Could you check a few things on this model? Use its own coordinates, in mm. A direction names the side the tool comes from. Round coordinates to 2 decimals unless told otherwise and drop trailing zeros. Order: outer loops, then holes, each group sorted by start corner. A loop starts at its lowest first (then second) coordinate and runs counter-clockwise, first axis right, second up. Notation, with made-up numbers: (68, 77.5) -> (106, 77.5) arc R17 ccw to (106, 103.5) -> close; hole circle Ø4 at (32.5, -29). An arc over 180 degrees is marked (long way). One line per question, with ' | ' between items.
Autodesk Inventor part; units mm, degrees
ref_plane "YZ Plane" through (0, 0, 0) normal (1, 0, 0) x (0, 1, 0)
ref_plane "XZ Plane" through (0, 0, 0) normal (0, 1, 0) x (-1, 0, 0)
ref_plane "XY Plane" through (0, 0, 0) normal (0, 0, 1) x (1, 0, 0)
sketch "Sketch1" plane through (0, 0, 0) normal (0, 1, 0) x (-1, 0, 0)
  line L0 (-24, 32.5) -> (24, 32.5)
  line L1 (24, 32.5) -> (24, -32.5)
  line L2 (24, -32.5) -> (-24, -32.5)
  line L3 (-24, -32.5) -> (-24, 32.5)
  line L4 (-24, 32.5) -> (24, -32.5) construction
  line L5 (24, 32.5) -> (-24, -32.5) construction
  line L6 (24, 9.5) -> (-24, 9.5)
  line L7 (-24, 9.5) -> (-24, -32.5)
  line L8 (-24, -32.5) -> (24, -32.5)
  line L9 (24, -32.5) -> (24, 9.5)
  circle A0 centre (0, -11.5) radius 11.25
  line L10 (24, 12.5) -> (-24, 12.5)
  line L11 (-24, 24.95) -> (-24, 20.05)
  line L12 (15.5, -27) -> (-15.5, -27) construction
  line L13 (-15.5, -27) -> (-15.5, 4) construction
  line L14 (-15.5, 4) -> (15.5, 4) construction
  line L15 (15.5, 4) -> (15.5, -27) construction
  line L16 (15.5, -27) -> (-15.5, 4) construction
  line L17 (-15.5, -27) -> (15.5, 4) construction
  line L18 (-24, 52.5) -> (24, 52.5)
  line L19 (24, 52.5) -> (24, 32.5)
  line L20 (24, 32.5) -> (-24, 32.5)
  line L21 (-24, 32.5) -> (-24, 52.5)
  point P0 (0, 0)
  point P1 (-21.1, 9.5)
  point P2 (21.1, 9.5)
  point P3 (18, 42.6936)
  point P4 (-11, 42.5)
  point P5 (18, 22.5)
  point P6 (-11, 22.3064)
  dimension "d0" = 48
  dimension "d1" = 65
  dimension "d2" = 20
  dimension "d3" = 3
  dimension "d4" = 2.9
  dimension "d5" = 2.9
  dimension "d6" = 22.5
  dimension "d35" = 31
  dimension "d36" = 31
  dimension "d71" = 20
  dimension "d73" = 6
  dimension "d74" = 6
  dimension "d82" = 35
  dimension "d83" = 35
extrude "Extrusion1" add sketch "Sketch1" along normal blind 4.2
sketch "Sketch2" plane through (0, 4.2, 0) normal (0, 1, 0) x (1, 0, 0)
  point P0 (0, 0)
  point P1 (11, -42.5)
  point P2 (11, -22.3064)
  point P3 (-18, -22.5)
  point P4 (-18, -42.6936)
hole "Hole5" at (11, 4.2, 42.5) at (-18, 4.2, 42.6936) at (11, 4.2, 22.3064) at (-18, 4.2, 22.5) direction (0, -1, 0) diameter 4.5 end through all
extrude "Extrusion3" add sketch "Sketch1" against normal blind 20 contours L1 L6 L3 L10
sketch "Sketch4" plane through (24, 0, -32.5) normal (1, 0, 0) x (0, 0, -1)
  line L0 (-42, -20) -> (-42, 0)
  line L1 (-42, -20) -> (-22, 0)
  line L2 (0, 0) -> (-42, 0)
  line L3 (-22, 0) -> (-42, 0)
  line L4 (-42, 0) -> (-42, -20)
  point P0 (-32.5, 0)
  dimension "d32" = 20
extrude "Extrusion4" add sketch "Sketch4" against normal blind 2.7
ref_plane "Work Plane1" through (0, 0, 52.5) normal (-1, 0, 0) x (0, 0, 1)
mirror "Mirror1" about plane through (0, 0, 52.5) normal (-1, 0, 0) of "Extrusion4"
sketch "Sketch5" plane through (0, 4.2, 0) normal (0, 1, 0) x (1, 0, 0)
  point P0 (0, 0)
  point P1 (-15.5, 27)
  point P2 (15.5, 27)
  point P3 (-15.5, -4)
  point P4 (15.5, -4)
hole "Hole4" at (-15.5, 4.2, -27) at (15.5, 4.2, -27) at (-15.5, 4.2, 4) at (15.5, 4.2, 4) direction (0, -1, 0) diameter 3.2 depth 8 tip angle 118 countersink diameter 6 countersink angle 90
sketch "Sketch6" plane through (21.3, -20, 9.5) normal (0, 0, -1) x (-1, 0, 0)
  line L0 (42.6, 0) -> (42.6, 20)
  line L1 (0, 20) -> (42.6, 20)
  line L2 (0, 20) -> (0, 0)
  line L3 (42.6, 0) -> (0, 0)
  point P0 (21.3, 20)
extrude "ajustement 0.2mm" cut sketch "Sketch6" against normal blind 0.4
sketch "Sketch7" plane through (0, 4.2, 0) normal (0, 1, 0) x (1, 0, 0)
  circle A0 centre (70.6822, -32.5) radius 55
  line L0 (21.3, -9.9) -> (-21.3, -9.9) construction
  line L1 (21.3, -9.9) -> (21.3, -51.2) construction
  line L2 (137, -22.5) -> (-72, -22.5) construction
  line L3 (0, -123.9517) -> (0, 131.2102) construction
  circle A1 centre (0, 11.5) radius 83.2585 construction
  line L4 (134.8387, -42.5) -> (-75.1613, -42.5) construction
  line L5 (134.8387, -32.5) -> (-75.1613, -32.5) construction
  point P0 (0, 0)
  dimension "d67" = 166.517
  dimension "d53" = 110
  dimension "d69" = 20
  dimension "d70" = 10
sketch "Sketch8" plane through (0, 0, 0) normal (0, -1, 0) x (1, 0, 0)
  line L0 (-21.3, 9.9) -> (21.3, 9.9)
  line L1 (21.3, -10.5) -> (21.3, 9.5)
  line L2 (-21.3, -10.5) -> (-21.3, 9.5)
  line L3 (21.3, 9.9) -> (-21.3, 9.9)
  line L4 (-18.3, 9.9) -> (-21.3, 6.9)
  line L5 (-21.3, 9.9) -> (-21.3, -10.5)
  line L6 (18.3, 9.9) -> (21.3, 6.9)
  line L7 (21.3, -10.5) -> (21.3, 9.9)
  point P0 (0, 0)
  dimension "d54" = 3
  dimension "d55" = 3
  dimension "d56" = 3
  dimension "d57" = 3
extrude "Extrusion6" add sketch "Sketch8" along normal blind 20
sketch "Sketch9" plane through (24, 0, -32.5) normal (1, 0, 0) x (0, 0, -1)
  line L0 (-39.4, -20) -> (-42, -20)
  line L1 (-39.4, -17.4) -> (-39.4, -20)
  line L2 (-42, -20) -> (-22, 0)
  point P0 (-32.5, 0)
extrude "Extrusion7" cut sketch "Sketch9" against normal through all
extrude "Extrusion8" cut sketch "Sketch7" against normal blind 30
sketch "Sketch10" plane through (-24, -20, 12.5) normal (0, 0, 1) x (1, 0, 0)
  line L0 (43.4475, 0) -> (43.4475, 20)
  line L1 (0, 20) -> (43.4475, 20)
  line L2 (0, 20) -> (0, 0)
  line L3 (43.4475, 0) -> (0, 0)
  point P0 (24, 20)
extrude "ajustement 0.2" cut sketch "Sketch10" against normal blind 0.2
equation "\"d55\" = d54"
equation "\"d56\" = d54"
equation "\"d57\" = d56"
properties part number "support_nema17_40mm"
1. I need wall thicknesses on probe 1 along Z at (x, y) = (-18, 1.3); probe 2 along X at (y, z) = (1.8, -27); probe 3 along Z at (x, y) = (15.5, 2). Which ranges of each line are inside material? Lowest first, please.
From the geometry:
probe 1: z = -32.5 to 20.25, 24.75 to 40.44, 44.94 to 52.5 | probe 2: x = -24 to -17.1, -13.9 to 13.9, 17.1 to 24 | probe 3: z = -32.5 to -28.6, -25.4 to 2.4, 5.6 to 52.5
2. I want a section at A-A on x = 0. List the corners of the cut face in (y, z) for me, and give its area (4 significant figures).
From the geometry:
outline: (-20, 9.9) -> (0, 9.9) -> (0, -0.25) -> (4.2, -0.25) -> (4.2, 52.5) -> (0, 52.5) -> (0, 12.3) -> (-20, 12.3) -> close; (0, -32.5) -> (4.2, -32.5) -> (4.2, -22.75) -> (0, -22.75) -> close | area: 310.5 mm²
3. On a 3-axis mill with a long thin cutter (end or side, diameter ignored), from which of +Z, -Z, +X, -X, +Y, -Y can I reach the whole of each face in a straight line? I mean faces 1 (the face through (21.3, -5, 2)), 2 (the face through (-17.086, 1.38, 3.792)), 3 (the face through (-3, -10, 12.3)). Say none if no direction works.
From the geometry:
face 1: -Z, -Y | face 2: +Y, -Y | face 3: +Z, -X, -Y
4. I want a section at D-D on y = -5. List the corners of the cut face in (x, z) for me, and give its area (3 significant figures).
From the geometry:
outline: (-24, -5.5) -> (-21.3, -5.5) -> (-21.3, 6.9) -> (-18.3, 9.9) -> (18.3, 9.9) -> (21.3, 6.9) -> (21.3, -5.5) -> (24, -5.5) -> (24, 3.42) arc R55 cw to (19.45, 12.5) -> (19.45, 12.3) -> (-24, 12.3) -> close | area: 186 mm²
5. If we mould it in two halves opening along Z, with no side actions, what happens to faces 4 (the face through (-19.8, -9.9, 8.4)), 5 (the face through (16.803, 0.336, 21.452)), 6 (the face through (-2, 2, 52.5))? For each: pulls with the +Z half, pulls with the -Z half, needs draft (parallel to the pull), parting line crosses it, or undercut.
From the geometry:
face 4: pulls with the -Z half | face 5: undercut | face 6: pulls with the +Z half
6. I'm going to push flat-ended pins straight in: pin 1 (4 mm diameter, centred on x = 15.5, z = -27, fed in from +Y); pin 2 (5 mm diameter, centred on x = -17.5, y = -16.5, fed in from +Z); pin 3 (7 mm diameter, centred on x = 11, z = 42.5, fed in from -Y). Where does each tip first touch, or does it pass through?
From the geometry:
pin 1: stops at y = 3.2 | pin 2: stops at z = 12.3 | pin 3: stops at y = 0
7. I want a section at C-C on y = -11. List the corners of the cut face in (x, z) for me.
From the geometry:
outline: (-24, 0.5) -> (-21.3, 0.5) -> (-21.3, 6.9) -> (-18.3, 9.9) -> (18.3, 9.9) -> (21.3, 6.9) -> (21.3, 0.5) -> (24, 0.5) -> (24, 3.42) arc R55 cw to (19.45, 12.5) -> (19.45, 12.3) -> (-24, 12.3) -> close
8. I want a section at B-B on z = -27. List the corners of the cut face in (x, y) for me, and give its area (3 significant figures).
From the geometry:
outline: (-24, 0) -> (-17.1, 0) -> (-17.1, 2.8) -> (-18.5, 4.2) -> (-24, 4.2) -> close; (-13.9, 0) -> (13.9, 0) -> (13.9, 2.8) -> (12.5, 4.2) -> (-12.5, 4.2) -> (-13.9, 2.8) -> close; (17.1, 0) -> (24, 0) -> (24, 4.2) -> (18.5, 4.2) -> (17.1, 2.8) -> close | area: 171 mm²
